CAD build for the part. Positions are in the model's coordinates, mm. Coordinates: 2 decimals unless noted, no trailing zeros. Loops run counter-clockwise (first coordinate to the right, second up) from the corner with the lowest first, then second, coordinate; pieces in that order, holes last.
1) Saw through at C-C, the plane z = 96. Write the cut outline in (x, y), and give its area (3 significant figures).
2) Saw through at A-A, the plane y = -6.5. Write the cut outline in (x, z), and give its area (3 significant figures).
3) Pin check, flat tip, straight feed: pin 1 Ø5.5 at (y, z) = (0, 64) entering from -X. Stop position of the tip, or through.
4) Wall check: line 1 along Y through (x, z) = (-7.75, 151); line 2 along Y through (x, z) = (-9.7, 96). Give the ranges that are in metal, low to high.
```python
from build123d import *

# Parameters (mm, degrees)
SKETCH1_W           = 18
SKETCH1_H           = 18
EXTRUDE_THIN1_DEPTH = 260
SKETCH2_R           = 3.4
CUT_EXTRUDE1_DEPTH  = 10


with BuildPart() as part:
    # Sketch1 → Extrude-Thin1 (new body)
    with BuildSketch(Plane.XY):
        with BuildLine():
            Line((-10, 9.5), (-10, -9.5))
            ThreePointArc((-10, -9.5), (-9.853553391, -9.853553391), (-9.5, -10))
            Line((-9.5, -10), (9.5, -10))
            ThreePointArc((9.5, -10), (9.853553391, -9.853553391), (10, -9.5))
            Line((10, -9.5), (10, 9.5))
            ThreePointArc((10, 9.5), (9.853553391, 9.853553391), (9.5, 10))
            Line((9.5, 10), (-9.5, 10))
            ThreePointArc((-9.5, 10), (-9.853553391, 9.853553391), (-10, 9.5))
        make_face()
        Rectangle(SKETCH1_W, SKETCH1_H, mode=Mode.SUBTRACT)
    extrude(amount=EXTRUDE_THIN1_DEPTH)

    # Sketch2 → Cut-Extrude1 (cut)
    with BuildSketch(Plane.ZY.offset(10)):
        with Locations((64, 0)):
            Circle(SKETCH2_R)
        with Locations((164, 0)):
            Circle(SKETCH2_R)
        with Locations((196, 0)):
            Circle(SKETCH2_R)
        with Locations((96, 0)):
            Circle(SKETCH2_R)
    extrude(amount=-CUT_EXTRUDE1_DEPTH, mode=Mode.SUBTRACT)


solid = part.part
```
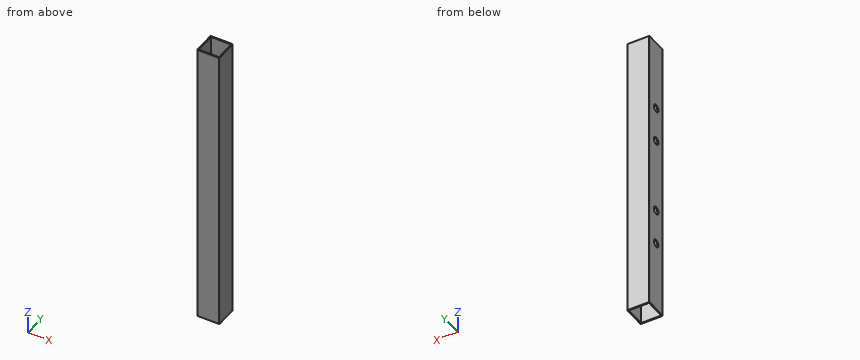
Data:
1. outline: (-10, -9.5) arc R0.5 ccw to (-9.5, -10) - (9.5, -10) arc R0.5 ccw to (10, -9.5) - (10, 9.5) arc R0.5 ccw to (9.5, 10) - (-9.5, 10) arc R0.5 ccw to (-10, 9.5) - (-10, 3.4) - (-9, 3.4) - (-9, 9) - (9, 9) - (9, -9) - (-9, -9) - (-9, -3.4) - (-10, -3.4) - close
1. area: 69.0 mm2
2. outline: (-10, 0) - (-9, 0) - (-9, 260) - (-10, 260) - close; (9, 0) - (10, 0) - (10, 260) - (9, 260) - close
2. area: 520 mm2
3. pin 1: stops at x = 9
4. line 1: y = -10 to -9, 9 to 10
4. line 2: y = -9.96 to -3.4, 3.4 to 9.96
